```python
from build123d import *

# Parameters (mm, degrees)
SKETCH_1_W                       = 42
SKETCH_1_H                       = 27
EXTRUDE_1_DEPTH                  = 2
SKETCH_2_W                       = 27
SKETCH_2_H                       = 30
SKETCH_2_W_2                     = 4
SKETCH_2_H_2                     = 5
EXTRUDE_2_DEPTH                  = 2
SKETCH_3_W                       = 4
SKETCH_3_H                       = 2.5
EXTRUDE_3_DEPTH                  = 2
SKETCH_4_R                       = 1.25
EXTRUDE_4_DEPTH                  = 2
PATTERN_LINEAR_1_COUNT           = 2
PATTERN_LINEAR_1_PITCH           = 16.5
PATTERN_LINEAR_1_COPY_1_SKETCH_R = 1.25
PATTERN_LINEAR_1_COPY_1_DEPTH    = 2
PATTERN_LINEAR_2_COUNT           = 2
PATTERN_LINEAR_2_PITCH           = 26.75
PATTERN_LINEAR_2_COPY_1_SKETCH_R = 1.25
PATTERN_LINEAR_2_COPY_1_DEPTH    = 2
FILLET_1_R                       = 4
SKETCH_8_R                       = 1.6
EXTRUDE_5_DEPTH                  = 2
MIRROR_4_COPY_1_SKETCH_R         = 1.6
MIRROR_4_COPY_1_DEPTH            = 2


with BuildPart() as part:
    # Эскиз1 → Бобышка-Вытянуть1 (new body)
    with BuildSketch(Plane(origin=(0, 0, 0), x_dir=(1, 0, 0), z_dir=(0, 1, 0))):
        Rectangle(SKETCH_1_W, SKETCH_1_H)
    extrude(amount=EXTRUDE_1_DEPTH)

    # Эскиз2 → Бобышка-Вытянуть2 (add)
    with BuildSketch(Plane(origin=(21, 0, 0), x_dir=(0, 0, -1), z_dir=(1, 0, 0))):
        with Locations((0, 17)):
            Rectangle(SKETCH_2_W, SKETCH_2_H)
        with Locations((-2.5, 6.5)):
            Rectangle(SKETCH_2_W_2, SKETCH_2_H_2, mode=Mode.SUBTRACT)
        with Locations((2.5, 16)):
            Rectangle(SKETCH_2_W_2, SKETCH_2_H_2, mode=Mode.SUBTRACT)
        with Locations((-2.5, 23)):
            Rectangle(SKETCH_2_W_2, SKETCH_2_H_2, mode=Mode.SUBTRACT)
    extrude_2 = extrude(amount=-EXTRUDE_2_DEPTH)

    # Зеркальное отражение1: Бобышка-Вытянуть2 across plane
    add(extrude_2.mirror(Plane(origin=(0, 0, 0), x_dir=(0, 0, 1), z_dir=(1, 0, 0))))

    # Эскиз3 → Бобышка-Вытянуть3 (add)
    with BuildSketch(Plane.ZY.offset(21)):
        with Locations((2.5, 24.25)):
            Rectangle(SKETCH_3_W, SKETCH_3_H)
        with Locations((-2.5, 17.25)):
            Rectangle(SKETCH_3_W, SKETCH_3_H)
        with Locations((2.5, 7.75)):
            Rectangle(SKETCH_3_W, SKETCH_3_H)
    extrude(amount=-EXTRUDE_3_DEPTH)

    # Эскиз4 → Бобышка-Вытянуть4 (add)
    with BuildSketch(Plane(origin=(0, 0, 13.5), x_dir=(-1, 0, 0), z_dir=(0, 0, -1))):
        with BuildLine():
            Line((-19, 9.5), (-19, 15.5))
            Line((-19, 15.5), (-12.5, 15.5))
            ThreePointArc((-12.5, 15.5), (-11.974953973, 15.270240895), (-11.5, 14.949489743))
            Line((-11.5, 14.949489743), (-11.5, 10.050510257))
            ThreePointArc((-11.5, 10.050510257), (-11.974953973, 9.729759105), (-12.5, 9.5))
            Line((-12.5, 9.5), (-19, 9.5))
        make_face()
        with Locations((-13.5, 12.5)):
            Circle(SKETCH_4_R, mode=Mode.SUBTRACT)
    extrude_4 = extrude(amount=EXTRUDE_4_DEPTH)

    # Зеркальное отражение2: Бобышка-Вытянуть4 across plane
    add(extrude_4.mirror(Plane(origin=(0, 0, 0), x_dir=(0, 0, 1), z_dir=(1, 0, 0))))

    # Линейный массив1: Бобышка-Вытянуть4 ×2
    with Locations(*[(0, i * PATTERN_LINEAR_1_PITCH, 0) for i in range(1, PATTERN_LINEAR_1_COUNT)]):
        add(extrude_4)

    # Линейный массив1 copy 1 sketch → Линейный массив1 copy 1 (add)
    with BuildSketch(Plane(origin=(0, 16.5, 13.5), x_dir=(1, 0, 0), z_dir=(0, 0, -1))):
        with BuildLine():
            Line((-19, -9.5), (-19, -15.5))
            Line((-19, -15.5), (-12.5, -15.5))
            ThreePointArc((-12.5, -15.5), (-11.974953973, -15.270240895), (-11.5, -14.949489743))
            Line((-11.5, -14.949489743), (-11.5, -10.050510257))
            ThreePointArc((-11.5, -10.050510257), (-11.974953973, -9.729759105), (-12.5, -9.5))
            Line((-12.5, -9.5), (-19, -9.5))
        make_face()
        with Locations((-13.5, -12.5)):
            Circle(PATTERN_LINEAR_1_COPY_1_SKETCH_R, mode=Mode.SUBTRACT)
    extrude(amount=PATTERN_LINEAR_1_COPY_1_DEPTH)

    # Линейный массив2: Бобышка-Вытянуть4 ×2
    with Locations(*[Vector(0, 0.3564269900834672, -0.9343231778887005) * (i * PATTERN_LINEAR_2_PITCH) for i in range(1, PATTERN_LINEAR_2_COUNT)]):
        add(extrude_4)

    # Линейный массив2 copy 1 sketch → Линейный массив2 copy 1 (add)
    with BuildSketch(Plane(origin=(0, 9.534421985, -11.493145009), x_dir=(1, 0, 0), z_dir=(0, 0, -1))):
        with BuildLine():
            Line((-19, -9.5), (-19, -15.5))
            Line((-19, -15.5), (-12.5, -15.5))
            ThreePointArc((-12.5, -15.5), (-11.974953973, -15.270240895), (-11.5, -14.949489743))
            Line((-11.5, -14.949489743), (-11.5, -10.050510257))
            ThreePointArc((-11.5, -10.050510257), (-11.974953973, -9.729759105), (-12.5, -9.5))
            Line((-12.5, -9.5), (-19, -9.5))
        make_face()
        with Locations((-13.5, -12.5)):
            Circle(PATTERN_LINEAR_2_COPY_1_SKETCH_R, mode=Mode.SUBTRACT)
    extrude(amount=PATTERN_LINEAR_2_COPY_1_DEPTH)

    # Скругление1
    fillet_1_edges = [part.edges().sort_by_distance(p)[0] for p in [
        (19, 15.5, 12.5),
        (19, 9.5, 12.5),
        (-19, 9.5, 12.5),
        (-19, 15.5, 12.5),
        (-19, 26, 12.5),
        (19, 26, 12.5),
        (-19, 19.034421985, -12.493145009),
        (-19, 25.034421985, -12.493145009),
        (19, 25.034421985, -12.493145009),
        (19, 19.034421985, -12.493145009),
    ]]
    fillet(fillet_1_edges, radius=FILLET_1_R)

    # Эскиз8 → Бобышка-Вытянуть5 (add)
    with BuildSketch(Plane(origin=(0, 0, 0), x_dir=(1, 0, 0), z_dir=(0, 1, 0))):
        with BuildLine():
            Line((-21, 13.5), (-18, 13.493145009))
            Line((-18, 13.493145009), (-15, 13.5))
            Line((-15, 13.5), (-15, 16.493145009))
            ThreePointArc((-15, 16.493145009), (-18, 22.098696284), (-21, 16.493145009))
            Line((-21, 16.493145009), (-21, 13.5))
        make_face()
        with Locations(Location((-18, 18.493145009, 0), (0, 0, 270))):
            Circle(SKETCH_8_R, mode=Mode.SUBTRACT)
    extrude_5 = extrude(amount=EXTRUDE_5_DEPTH)

    # Зеркальное отражение3: Бобышка-Вытянуть5 across plane
    add(extrude_5.mirror(Plane(origin=(0, 0, 0), x_dir=(0, 0, 1), z_dir=(1, 0, 0))))

    # Зеркальное отражение4: Бобышка-Вытянуть5 across plane
    add(extrude_5.mirror(Plane.XY))

    # Зеркальное отражение4 copy 1 sketch → Зеркальное отражение4 copy 1 (add)
    with BuildSketch(Plane(origin=(0, 0, 0), x_dir=(-1, 0, 0), z_dir=(0, 1, 0))):
        with BuildLine():
            Line((-21, 13.5), (-18, 13.493145009))
            Line((-18, 13.493145009), (-15, 13.5))
            Line((-15, 13.5), (-15, 16.493145009))
            ThreePointArc((-15, 16.493145009), (-18, 22.098696284), (-21, 16.493145009))
            Line((-21, 16.493145009), (-21, 13.5))
        make_face()
        with Locations(Location((-18, 18.493145009, 0), (0, 0, 270))):
            Circle(MIRROR_4_COPY_1_SKETCH_R, mode=Mode.SUBTRACT)
    extrude(amount=MIRROR_4_COPY_1_DEPTH)


solid = part.part
```
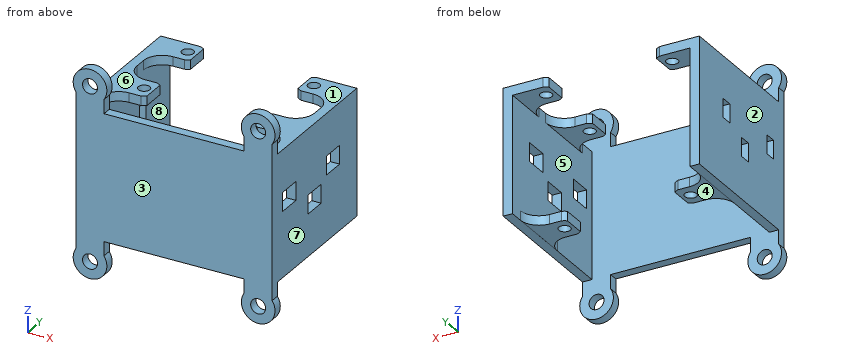
Read the model definition and answer for the solid it produces. Units are mm, in the model's axes. Face numbers are marked on the shaded views. A direction names the side the tool comes from. Coordinates: 2 decimals unless noted, no trailing zeros. Write each loop counter-clockwise with the first axis right and the second up, starting at its lowest first coordinate (ties: lowest second). Pieces come first, ordered by that corner, then holes. Notation, with made-up numbers: (-26, 18) -> (-6, 18) arc R25 ccw to (-6, 30) -> close; hole circle Ø1 at (-4.75, -4.75). An arc over 180 degrees is marked (long way). Write item = value, one per line.
(1) Given pin 1 Ø10 at (x, z) = (-3, -16) entering from +Y; pin 2 Ø12 at (y, z) = (20.5, 10) entering from -X; pin 3 Ø0.6 at (x, y) = (-20, 22) entering from +Z, each flat-ended and moving along its own axis, determine where each tip first touches the part or whether it passes through.
From the geometry:
pin_1 = 2
pin_2 = -21
pin_3 = 13.5
(2) Section C-C on y = 12.5 is taken. Write down the section's boundary in (x, z).
From the geometry:
outline = (-21, -13.5) -> (-19, -13.5) -> (-19, 11.5) -> (-14.75, 11.5) -> (-14.75, 13.5) -> (-21, 13.5) -> close; (-12.25, 11.5) -> (-11.5, 11.5) -> (-11.5, 13.5) -> (-12.25, 13.5) -> close; (11.5, 11.5) -> (12.25, 11.5) -> (12.25, 13.5) -> (11.5, 13.5) -> close; (14.75, 11.5) -> (19, 11.5) -> (19, -13.5) -> (21, -13.5) -> (21, 13.5) -> (14.75, 13.5) -> close
(3) Section B-B on z = -15.5 is taken. Write down the section's boundary in (x, y), plus the area to 3 significant figures.
From the geometry:
outline = (-21, 0) -> (-15, 0) -> (-15, 2) -> (-21, 2) -> close; (15, 0) -> (21, 0) -> (21, 2) -> (15, 2) -> close
area = 24.0 mm2
(4) Section D-D on z = 3.5 is taken. Write down the section's boundary in (x, y).
From the geometry:
outline = (-21, 0) -> (21, 0) -> (21, 4) -> (19, 4) -> (19, 2) -> (-19, 2) -> (-19, 4) -> (-21, 4) -> close; (-21, 6.5) -> (-19, 6.5) -> (-19, 20.5) -> (-21, 20.5) -> close; (-21, 23) -> (-19, 23) -> (-19, 32) -> (-21, 32) -> close; (19, 9) -> (21, 9) -> (21, 20.5) -> (19, 20.5) -> close; (19, 25.5) -> (21, 25.5) -> (21, 32) -> (19, 32) -> close
(5) Straight lines are drawn through the part: L1, parallel to Y at x = -13.5, z = 12.9; L2, parallel to Y at x = -13.5, z = -12.05; L3, parallel to X at y = 13.5, z = 13. For each, find the intervals that lie inside material, in ascending order. Write a range as from..to.
From the geometry:
L1 = 0..2, 9.5..11.25, 13.75..15.5, 26..27.75, 30.25..32
L2 = 0..2, 19.03..20.78, 23.28..25.03
L3 = -21..-14.25, -12.75..-11.5, 11.5..12.75, 14.25..21
(6) For a pull along X with two mould halves and no side action, classify the marked faces 5, 6, 7 and 8 as +X half, -X half, draft (parallel to the pull), parting line (faces both ways), or undercut.
From the geometry:
face_5 = undercut
face_6 = draft
face_7 = +X half
face_8 = undercut
(7) Which of the six approach directions +Z, -Z, +X, -X, +Y, -Y give full straight-line access (tool end or side, diameter ignored) to the marked faces 1, 2, 3 and 4?
From the geometry:
face_1 = +Z, +X, -X, +Y
face_2 = -X, +Y, -Y
face_3 = +Z, -Z, +X, -X, -Y
face_4 = -Z, +X, -X, +Y
(8) Section A-A on x = 13.5 is taken. Write down the section's boundary in (y, z), plus the area to 3 significant figures.
From the geometry:
outline = (0, -13.5) -> (2, -13.5) -> (2, 13.5) -> (0, 13.5) -> close; (9.5, 11.5) -> (11.25, 11.5) -> (11.25, 13.5) -> (9.5, 13.5) -> close; (13.75, 11.5) -> (15.5, 11.5) -> (15.5, 13.5) -> (13.75, 13.5) -> close; (19.03, -13.49) -> (20.78, -13.49) -> (20.78, -11.49) -> (19.03, -11.49) -> close; (23.28, -13.49) -> (25.03, -13.49) -> (25.03, -11.49) -> (23.28, -11.49) -> close; (26, 11.5) -> (27.75, 11.5) -> (27.75, 13.5) -> (26, 13.5) -> close; (30.25, 11.5) -> (32, 11.5) -> (32, 13.5) -> (30.25, 13.5) -> close
area = 75.0 mm2
